from build123d import *

# Parameters (mm, degrees)
F0_R          = 24.13
F0_R_2        = 20.447
F1_DEPTH      = 1308.1
F3_DEPTH      = 24.131
F3_DEPTH_BACK = 24.131
F5_DEPTH      = 24.131
F5_DEPTH_BACK = 24.131
F8_W          = 230.4114792496
F8_H          = 177.8236068785
F9_DEPTH      = 25.4
F9_DEPTH_BACK = 20.32


with BuildPart() as f1:
    # F0 (on Top) → F1 (new body)
    with BuildSketch(Plane.XY):
        Circle(F0_R)
        Circle(F0_R_2, mode=Mode.SUBTRACT)
    extrude(amount=F1_DEPTH)

    # F2 (on Right) → F3 (cut, two sides)
    with BuildSketch(Plane.YZ) as f3_sk:
        Polygon((24.13, 1288.3563127231), (24.13, 1308.1), (-24.13, 1308.1), align=None)
    extrude(amount=-F3_DEPTH, mode=Mode.SUBTRACT)
    extrude(f3_sk.sketch, amount=F3_DEPTH_BACK, mode=Mode.SUBTRACT)

    # F4 (on Front) → F5 (cut, two sides)
    with BuildSketch(Plane.XZ) as f5_sk:
        Polygon((-28.575, 0), (28.575, 0), (28.575, 26.6494826636), align=None)
    extrude(amount=F5_DEPTH, mode=Mode.SUBTRACT)
    extrude(f5_sk.sketch, amount=-F5_DEPTH_BACK, mode=Mode.SUBTRACT)

    # F8 (on line) → F9 (cut, two sides)
    with BuildSketch(Plane(origin=(-2.5518360133, -6.0381584146, 5.4724299905), x_dir=(-0.9543044076, 0.2214273865, -0.2006813646), z_dir=(0.2988362387, 0.7071067812, -0.6408563821))) as f9_sk:
        with Locations((9.1961668804, 17.1195510775)):
            Rectangle(F8_W, F8_H)
    extrude(amount=F9_DEPTH, mode=Mode.SUBTRACT)
    extrude(f9_sk.sketch, amount=-F9_DEPTH_BACK, mode=Mode.SUBTRACT)


solid = f1.part
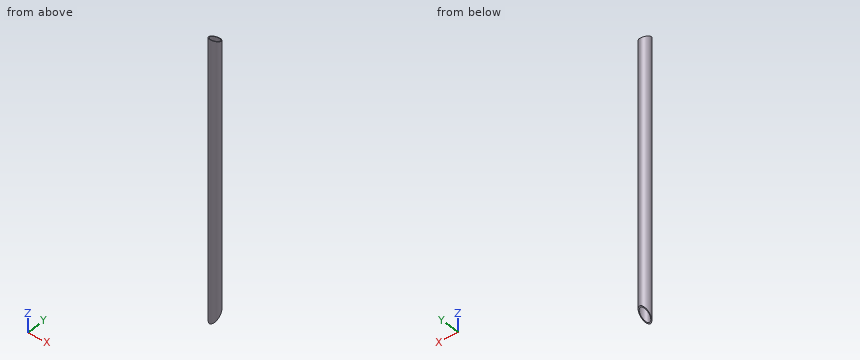
Geometry check sheet. Reference: the model listing, model coordinates, mm. Round coordinates to 2 decimals unless told otherwise and drop trailing zeros. Order: outer loops, then holes, each group sorted by start corner. A loop starts at its lowest first (then second) coordinate and runs counter-clockwise, first axis right, second up. Notation, with made-up numbers: (-6.75, 60) -> (-0.75, 60) arc R25 ccw to (-0.75, 90) -> close; hole circle Ø5 at (36.25, 14). An arc over 180 degrees is marked (long way). Use one line per item in the form item = value.
1. Cross-section at C-C, the plane z = 314. Enter the section's corners in (x, y), plus the area to 3 significant figures.
Working result:
outline = circle Ø48.26 at (0, 0); hole circle Ø40.89 at (0, 0)
area = 516 mm^2
2. Go/stop test with flat-tipped pins: pin 1 (3 mm diameter, centred on x = -15.5, z = 528, fed in from -Y); pin 2 (8 mm diameter, centred on y = 4.5, z = 915, fed in from -X); pin 3 (6 mm diameter, centred on x = -17.5, z = 323, fed in from +Y). Record where each tip stops, or that it passes through.
Working result:
pin_1 = -19.65
pin_2 = -24.12
pin_3 = 19.29
3. Cross-section at B-B, the plane x = 0. Enter the section's corners in (y, z).
Working result:
outline = (-24.13, 18.41) -> (-20.45, 22.47) -> (-20.45, 1306.59) -> (-24.13, 1308.1) -> close; (20.45, 67.59) -> (24.13, 71.66) -> (24.13, 1288.36) -> (20.45, 1289.86) -> close
4. Scan lines: line 1 along X through (y, z) = (3, 161); line 2 along X through (y, z) = (0, 705). Record each from-to range of solid material in increasing order. Write a range as from..to.
Working result:
line_1 = -23.94..-20.23, 20.23..23.94
line_2 = -24.13..-20.45, 20.45..24.13
5. Cross-section at A-A, the plane y = -12. Enter the section's corners in (x, z), plus the area to 3 significant figures.
Working result:
outline = (-20.93, 22.03) -> (-16.56, 24.07) -> (-16.56, 1303.14) -> (-20.93, 1303.14) -> close; (16.56, 39.51) -> (20.93, 41.55) -> (20.93, 1303.14) -> (16.56, 1303.14) -> close
area = 11,100 mm^2
